Model file for the job. Use its own axes, mm. Face numbers are marked on the shaded views. A direction names the side the tool comes from. Coordinates: 2 decimals unless noted, no trailing zeros. Write each loop counter-clockwise with the first axis right and the second up, starting at its lowest first coordinate (ties: lowest second). Pieces come first, ordered by that corner, then holes.
Q1. Band-saw the part on D-D, the plane x = -55. Write the cut outline in (y, z).
Q2. Pin check, flat tips, straight feed: P1, Ø4.5, axis at x = -31.82, y = 31.82, coming from the +Z side; P2, Ø8, axis at x = -7, z = 19.5, coming from the +Y side; P3, Ø10, axis at y = -49, z = 23.5, coming from the +X side; P4, Ø6, axis at y = -47.5, z = 26.5, coming from the +X side. Stop position of each tip, or through.
Q3. Band-saw the part on A-A, the plane x = 52. Write the cut outline in (y, z).
Q4. Which spindle directions (+Z, -Z, +X, -X, +Y, -Y) get a long thin tool onto all of the face, cutting with end or side? Do the marked faces 5 and 6. Say none if no direction does.
Q5. Band-saw the part on B-B, the plane z = 15.5. State how many separate pieces and enclosed holes the cut face has, plus the area to 3 significant figures.
Q6. Pull direction Y, two halves, no side cores. Call the marked faces 1, 2, 3 and 4: released by +Y, released by -Y, zero draft, split by the parting line, or undercut.
Q7. Drill centre lines: probe 1 along Y at (x, z) = (34, 15.5); probe 2 along Y at (x, z) = (-33, 15.5); probe 3 along Z at (x, y) = (14, 6). Where is each one in solid material? Low to high.
from build123d import *

# Parameters (mm, degrees)
SKETCH3_R          = 65
SKETCH3_R_2        = 2.75
EXTRUDE1_DEPTH     = 34
CUT_EXTRUDE2_DEPTH = 20
SKETCH22_R         = 6.8
CUT_EXTRUDE3_DEPTH = 53.960179098
SKETCH26_R         = 9
CUT_EXTRUDE4_DEPTH = 35.0000001
SKETCH27_R         = 9
CUT_EXTRUDE5_DEPTH = 36.160179098


with BuildPart() as part:
    # Sketch3 → Extrude1 (new body)
    with BuildSketch(Plane.XY):
        Circle(SKETCH3_R)
        with Locations((31.819805153, -31.819805153)):
            Circle(SKETCH3_R_2, mode=Mode.SUBTRACT)
        with Locations((-31.819805153, -31.819805153)):
            Circle(SKETCH3_R_2, mode=Mode.SUBTRACT)
        with Locations((31.819805153, 31.819805153)):
            Circle(SKETCH3_R_2, mode=Mode.SUBTRACT)
        with Locations((-31.819805153, 31.819805153)):
            Circle(SKETCH3_R_2, mode=Mode.SUBTRACT)
    extrude(amount=EXTRUDE1_DEPTH)

    # Sketch3_6 → Cut-Extrude2 (cut)
    with BuildSketch(Plane.XY):
        with BuildLine():
            Line((-20.421328258, 43.144950309), (-27.237880936, 26.740610009))
            ThreePointArc((-27.237880936, 26.740610009), (-28.54324707, 23.999538948), (-30.118972052, 21.404439318))
            add(Edge.make_bspline(
                [(-8.411618966, 31.392589354), (-6.594986557, 31.927343906), (-4.727596656, 32.304011663), (-0.947579394, 32.726950043), (0.964989801, 32.773208373), (4.777108777, 32.531081057), (6.676598891, 32.242693441), (10.404207822, 31.337263886), (12.232267294, 30.720230446), (15.760360448, 29.173637758), (17.460336939, 28.244097303), (20.679062247, 26.098347596), (22.197757805, 24.882166939), (25.005835643, 22.198009273), (26.295170268, 20.730069861), (28.60307704, 17.585286262), (29.621608652, 15.90848759), (31.354425209, 12.395644964), (32.068678043, 10.559653108), (33.168512452, 6.783381836), (33.554071399, 4.84315955), (33.981977998, 0.91703866), (34.024313279, -1.068799499), (33.761644813, -5.025657895), (33.456639413, -6.996616206), (32.505786005, -10.863180522), (31.859947203, -12.758725015), (30.244434466, -16.415746217), (29.274780398, -18.177163724), (27.038718465, -21.510852538), (25.772340603, -23.083068793), (22.979235835, -25.988634722), (21.452548225, -27.321935222), (18.18350905, -29.706877352), (16.441204938, -30.758477245), (12.792592203, -32.545523582), (10.886337796, -33.28093707), (6.966927518, -34.410539179), (4.95383101, -34.804704707), (0.881572969, -35.237007362), (-1.17752584, -35.275132047), (-5.279057127, -34.991353155), (-7.321425423, -34.669448256), (-11.326780574, -33.672621975), (-13.289703752, -32.997710517), (-17.075395447, -31.312765708), (-18.898102754, -30.302753307), (-22.346412369, -27.975919739), (-23.971957836, -26.659129989), (-26.974594454, -23.756685335), (-28.351634915, -22.171071432), (-30.813133029, -18.777462502), (-31.89754775, -16.969516871), (-33.738297145, -13.184908034), (-34.494598024, -11.208301165), (-35.653409825, -7.145620969), (-36.055897198, -5.05960924), (-36.492023631, -0.841182208), (-36.525650191, 1.29116809), (-36.220191785, 5.537304064), (-35.881105833, 7.651023301), (-34.837758132, 11.795003117), (-34.13350703, 13.825197856), (-32.378618873, 17.739300975), (-31.328003859, 19.623146143), (-30.118972052, 21.404439318)],
                knots=[0, 0, 0, 0, 0.03125, 0.03125, 0.0625, 0.0625, 0.09375, 0.09375, 0.125, 0.125, 0.15625, 0.15625, 0.1875, 0.1875, 0.21875, 0.21875, 0.25, 0.25, 0.28125, 0.28125, 0.3125, 0.3125, 0.34375, 0.34375, 0.375, 0.375, 0.40625, 0.40625, 0.4375, 0.4375, 0.46875, 0.46875, 0.5, 0.5, 0.53125, 0.53125, 0.5625, 0.5625, 0.59375, 0.59375, 0.625, 0.625, 0.65625, 0.65625, 0.6875, 0.6875, 0.71875, 0.71875, 0.75, 0.75, 0.78125, 0.78125, 0.8125, 0.8125, 0.84375, 0.84375, 0.875, 0.875, 0.90625, 0.90625, 0.9375, 0.9375, 0.96875, 0.96875, 1, 1, 1, 1], degree=3))
            Line((-8.411618966, 31.392589354), (-6.015539335, 37.158862647))
            Line((-6.015539335, 37.158862647), (-20.421328258, 43.144950309))
        make_face()
    extrude(amount=CUT_EXTRUDE2_DEPTH, mode=Mode.SUBTRACT)

    # Sketch22 → Cut-Extrude3 (cut, through all)
    with BuildSketch(Plane(origin=(12.281446339, 29.555852442, 0), x_dir=(-0.923448008, 0.383723568, 0), z_dir=(0.383723568, 0.923448008, 0))):
        with Locations(Location((27.613769175, 12, 0), (0, 0, 180))):  # turned: the seam where the file's is
            Circle(SKETCH22_R)
    extrude(amount=CUT_EXTRUDE3_DEPTH, mode=Mode.SUBTRACT)

    # Sketch26 → Cut-Extrude4 (cut, through all)
    with BuildSketch(Plane.XY):
        Circle(SKETCH26_R)
    extrude(amount=CUT_EXTRUDE4_DEPTH, mode=Mode.SUBTRACT)

    # Sketch27 → Cut-Extrude5 (cut, through all)
    with BuildSketch(Plane(origin=(19.11172585, 45.993226983, 0), x_dir=(0.923448008, -0.383723568, 0), z_dir=(-0.383723568, -0.923448008, 0))):
        with Locations((-27.613769175, 12)):
            Circle(SKETCH27_R)
    extrude(amount=-CUT_EXTRUDE5_DEPTH, mode=Mode.SUBTRACT)


solid = part.part
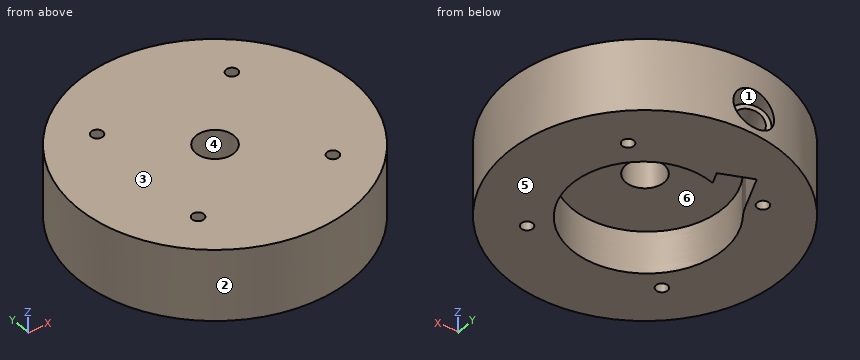
Answer sheet:
1. outline: (-34.64, 0) - (34.64, 0) - (34.64, 34) - (-34.64, 34) - close
2. P1: passes through
2. P2: stops at y = 64.92
2. P3: stops at x = 47.84
2. P4: stops at x = 47.38
3. outline: (-39, 0) - (39, 0) - (39, 34) - (-39, 34) - close
4. face 5: -Z, +X, -X, +Y, -Y
4. face 6: -Z
5. separate pieces: 1
5. enclosed holes: 4
5. area: 8,840 mm2
6. face 1: undercut
6. face 2: split by the parting line
6. face 3: zero draft
6. face 4: undercut
7. probe 1: y = -55.4 to -33.5, -30.14 to 30.14, 33.5 to 55.4
7. probe 2: y = -56 to -34.3, -29.34 to -14.7, 16.34 to 29.34, 34.3 to 56
7. probe 3: z = 20 to 34
